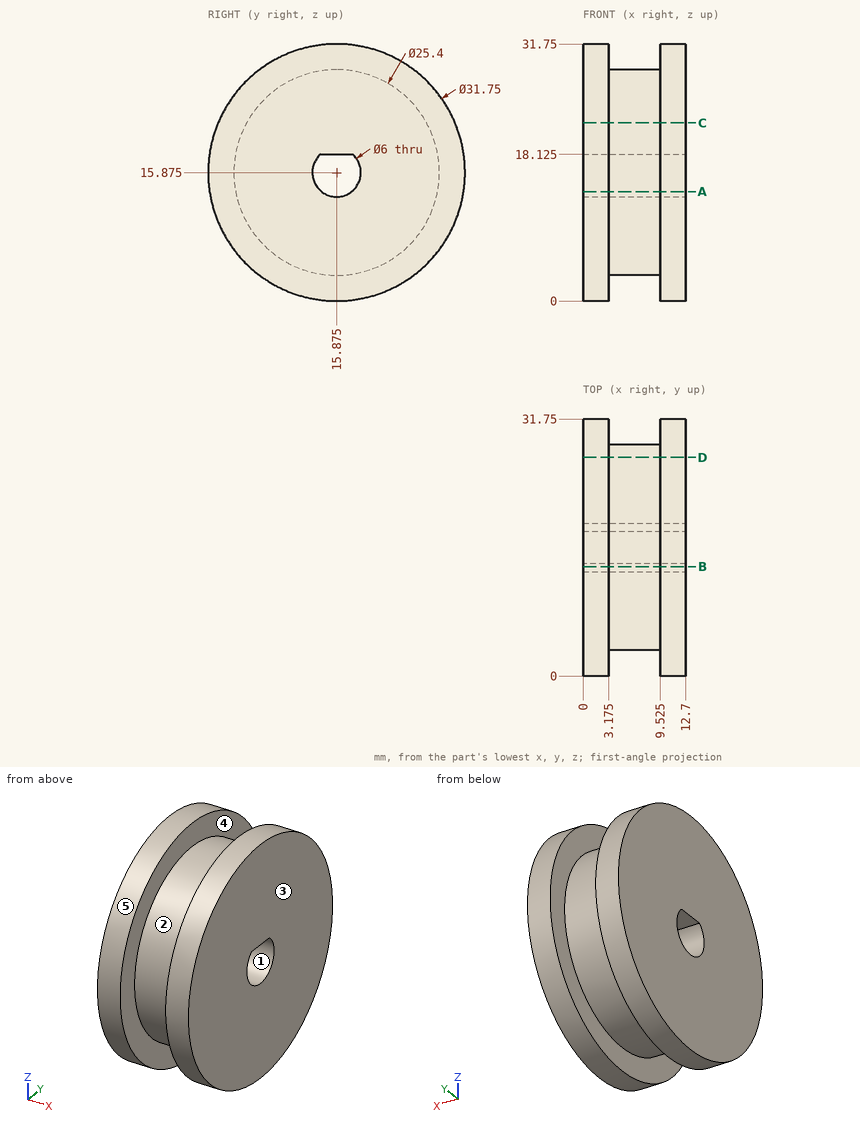
Answer from the drawing. Dimensions are ordinates in mm from the lowest x, y and z of the part. A direction names the side the tool comes from. Round coordinates to 2 decimals unless told otherwise and drop trailing zeros. Write each loop counter-clockwise with the first axis right and the second up, starting at its lowest first coordinate (ties: lowest second). Pieces come first, ordered by that corner, then holes.
1. The part is cut by section D-D, the plane y = 27. Determine the outline of the cut face in (x, z) (3 decimals).
2. Straight lines are drawn through the part: L1, parallel to X at y = 10, z = 3.5 (3 decimals); L2, parallel to Z at x = 2.5, y = 16 (1 decimal); L3, parallel to Z at x = 7, y = 18.5. For each, find the intervals that lie inside material, in ascending order.
3. The part is cut by section A-A, the plane z = 13.5. Determine the outline of the cut face in (x, y) (3 decimals).
4. Which of the six approach directions +Z, -Z, +X, -X, +Y, -Y give full straight-line access (tool end or side, diameter ignored) to the marked faces 1 and 2?
5. The part is cut by section C-C, the plane z = 22. Determine the outline of the cut face in (x, y) (3 decimals).
6. Given pin 1 Ø1.5 at (x, z) = (4.5, 11) entering from +Y; pin 2 Ø5 at (x, y) = (10, 4.5) entering from -Z; pin 3 Ø6 at (x, z) = (2, 12) entering from -Y, each flat-ended and moving along its own axis, determine where each tip first touches the part or whether it passes through.
7. Determine the mould class of the marked faces 3, 4 and 5 for opening direction X: pulls with the +X half, pulls with the -X half, needs draft (parallel to the pull), parting line crosses it, or undercut.
Values:
1. outline: (0, 4.55) - (3.175, 4.55) - (3.175, 9.749) - (9.525, 9.749) - (9.525, 4.55) - (12.7, 4.55) - (12.7, 27.2) - (9.525, 27.2) - (9.525, 22.001) - (3.175, 22.001) - (3.175, 27.2) - (0, 27.2) - close
2. L1: x = 0 to 3.175, 9.525 to 12.7
2. L2: z = 0 to 12.9, 18.1 to 31.7
2. L3: z = 3.45 to 14.42, 17.33 to 28.3
3. outline: (0, 0.179) - (3.175, 0.179) - (3.175, 3.399) - (9.525, 3.399) - (9.525, 0.179) - (12.7, 0.179) - (12.7, 14.042) - (0, 14.042) - close; (0, 17.708) - (12.7, 17.708) - (12.7, 31.571) - (9.525, 31.571) - (9.525, 28.351) - (3.175, 28.351) - (3.175, 31.571) - (0, 31.571) - close
4. face 1: +X, -X
4. face 2: none
5. outline: (0, 1.229) - (3.175, 1.229) - (3.175, 4.75) - (9.525, 4.75) - (9.525, 1.229) - (12.7, 1.229) - (12.7, 30.521) - (9.525, 30.521) - (9.525, 27) - (3.175, 27) - (3.175, 30.521) - (0, 30.521) - close
6. pin 1: stops at y = 27.89
6. pin 2: stops at z = 2.71
6. pin 3: stops at y = 0.02
7. face 3: pulls with the +X half
7. face 4: undercut
7. face 5: needs draft
